```python
from build123d import *

# Parameters (mm, degrees)
ESQUISSE1_R                               = 37.5
BOSS_EXTRU_1_DEPTH                        = 5
TROU_POUR_TARAUDAGE_POUR_TROU_TARAUD_M5_D = 4.2
R_P_TITION_CIRCULAIRE1_COUNT              = 4
BOSS_EXTRU_2_DEPTH                        = 5
TROU_POUR_TARAUDAGE_POUR_TROU_TARAUD_2_D  = 4.2


with BuildPart() as part:
    # Esquisse1 → Boss.-Extru.1 (new body)
    with BuildSketch(Plane.XY):
        Circle(ESQUISSE1_R)
    extrude(amount=BOSS_EXTRU_1_DEPTH)

    # Trou pour taraudage pour trou taraud_ M5 (through all)
    with Locations(Plane.XY.offset(5)):
        with Locations((3.3162691, -29.816142595)):
            trou_pour_taraudage_pour_trou_taraud_m5 = Hole(TROU_POUR_TARAUDAGE_POUR_TROU_TARAUD_M5_D / 2)

    # Répétition circulaire1: Trou pour taraudage pour trou taraud_ M5 ×4 about axis
    r_p_tition_circulaire1_axis = Axis((0, 0, 0), (0, 0, 1))
    for i in range(1, R_P_TITION_CIRCULAIRE1_COUNT):
        add(trou_pour_taraudage_pour_trou_taraud_m5.rotate(r_p_tition_circulaire1_axis, i * 360 / R_P_TITION_CIRCULAIRE1_COUNT), mode=Mode.SUBTRACT)

    # Esquisse4 → Boss.-Extru.2 (add)
    with BuildSketch(Plane.XY.offset(5)):
        with BuildLine():
            ThreePointArc((-55.427721141, -2.370238342), (-63.3788401, -14.426455821), (-50.992891265, -21.853497228))
            add(Edge.make_bspline(
                [(-27.47890369, -25.517833999), (-30.318179528, -22.460357126), (-38.333660049, -19.857417418), (-46.174070418, -20.537027691), (-50.992891265, -21.853497228)],
                knots=[0, 0, 0, 0, 0.450210397, 1, 1, 1, 1], degree=3))
            ThreePointArc((-27.47890369, -25.517833999), (-36.564715442, -8.322955281), (-35.816319782, 11.110411212))
            add(Edge.make_bspline(
                [(-35.816319782, 11.110411212), (-37.052534505, 7.125260617), (-43.151729094, 1.309501984), (-50.513854322, -1.471328291), (-55.427721141, -2.370238342)],
                knots=[0, 0, 0, 0, 0.450210397, 1, 1, 1, 1], degree=3))
        make_face()
    extrude(amount=-BOSS_EXTRU_2_DEPTH)

    # Trou pour taraudage pour trou taraud 2 (through all)
    with Locations(Plane.XY.offset(5)):
        with Locations((-53.628249316, -12.207001079)):
            Hole(TROU_POUR_TARAUDAGE_POUR_TROU_TARAUD_2_D / 2)


solid = part.part
```
CAD build for the part. Positions are in the model's coordinates, mm. Give positions to 0.01 mm unless a question says otherwise; leave off trailing zeros. Loops run counter-clockwise (first coordinate to the right, second up) from the corner with the lowest first, then second, coordinate; pieces in that order, holes last. Notation, with made-up numbers: M 32,-11.75 L 46,-11.75 A20 ccw 46,20.25 Z; hole C 61,-33.75 d6. An arc over 180 degrees is marked long. Use one line per item in the form item = value.
Item 1: Two-plate mould, pull along Y, no slides. Class faces 1 (the face through (36.845, 6.978, 2.465)), 2 (the face through (-3, 1, 0)), 3 (the face through (-31.866, -3.772, 2.465)): pulls with the +Y half, pulls with the -Y half, needs draft (parallel to the pull), parting line crosses it, or undercut.
Determined:
face_1 = parting line crosses it
face_2 = needs draft
face_3 = undercut
Item 2: Flat gauge pins, fed straight in: pin 1 (1 mm diameter, centred on x = -38, z = 2, fed in from -Y); pin 2 (5.5 mm diameter, centred on x = -3.32, y = 29.82, fed in from -Z); pin 3 (2 mm diameter, centred on y = 15, z = 2.5, fed in from +X); pin 4 (2 mm diameter, centred on x = 0.5, z = 1.5, fed in from +Y). Where does each tip first touch, or does it go through?
Determined:
pin_1 = -20.78
pin_2 = 0
pin_3 = 34.79
pin_4 = 37.5
Item 3: Drill centre lines: probe 1 along X at (y, z) = (-14, 4.1); probe 2 along X at (y, z) = (-11, 4.4); probe 3 along Y at (x, z) = (28, 3.9). Where is each one in solid material? Low to high. Write a range as from..to.
Determined:
probe_1 = -63.47..-54.72, -52.54..34.79
probe_2 = -63.56..-55.35, -51.91..35.85
probe_3 = -24.94..2.26, 4.37..24.94
Item 4: Slice it at A-A (y = 12.5). List the corners of the cut face in (x, z), plus the area to 3 significant figures.
Determined:
outline = M -35.36,0 L 35.36,0 L 35.36,5 L -35.36,5 Z
area = 354 mm2
Item 5: Slice it at C-C (z = 3.6). Count the separate pieces of the cut face and the enclosed holes in it, plus the area to 3 significant figures.
Determined:
separate_pieces = 1
enclosed_holes = 5
area = 4,920 mm2
Item 6: Slice it at B-B (x = -10). List the corners of the cut face in (y, z).
Determined:
outline = M -36.14,0 L 36.14,0 L 36.14,5 L -36.14,5 Z
